Build history of the part. All positions in model axes, mm. Face numbers are marked on the shaded views. A direction names the side the tool comes from. Round coordinates to 2 decimals unless told otherwise and drop trailing zeros. Write each loop counter-clockwise with the first axis right and the second up, starting at its lowest first coordinate (ties: lowest second). Pieces come first, ordered by that corner, then holes. Notation, with made-up numbers: (-20.5, -14) - (0.5, -14) arc R30 ccw to (0.5, 9) - close; hole circle Ø11 at (46, 30.5). An arc over 180 degrees is marked (long way). One line per question, with ' | ' between items.
from build123d import *

# Parameters (mm, degrees)
F1_DEPTH = 76.2
F3_DEPTH = 25.4
F5_DEPTH = 49.022
F6_R     = 15.3034000689
F6_R_2   = 10.835787307
F6_R_3   = 5.9493654503
F7_DEPTH = 25.4
F8_DEPTH = 12.7
F9_DEPTH = 120.396


# Not quite as in the source:
# - a fillet or chamfer that OpenCascade refuses, or shapes differently, is made with other operations: its cross-section is extruded or revolved along the edge and cut away or added


with BuildPart() as f1:
    # F0 (on Front) → F1 (new body)
    with BuildSketch(Plane.XZ):
        Polygon((43.6695814133, 73.2915997505), (0, 0), (-37.7974100411, 0), (-75.9054422379, 48.224221915), (-75.9054422379, -55.3548447788), (43.6695814133, -55.3548447788), align=None)
    extrude(amount=F1_DEPTH)

    # F2 (on face) → F3 (join)
    with BuildSketch(Plane.XZ.offset(76.2)):
        Polygon((43.6695814133, 73.2915997505), (0, 0), (0, -55.3548447788), (43.6695814133, -55.3548447788), align=None)
    extrude(amount=F3_DEPTH)

    # F4 (on face) → F5 (cut)
    with BuildSketch(Plane.XZ.offset(76.2)):
        Polygon((-75.9054422379, 0), (-37.7974100411, 0), (-75.9054422379, 48.224221915), align=None)
    extrude(amount=-F5_DEPTH, mode=Mode.SUBTRACT)

    # F6 (on face) → F7 (join)
    with BuildSketch(Plane.XY):
        with Locations((-18.1702096015, -18.0441774428)):
            Circle(F6_R)
        with Locations((-44.1785492003, -40.8460125327)):
            Circle(F6_R_2)
        with Locations((-63.5862797499, -57.4966222048)):
            Circle(F6_R_3)
    extrude(amount=F7_DEPTH)

    # F8 (cut): a face of the model
    f8_faces = [f1.faces().sort_by_distance(p)[0] for p in [
        (-56.8514261395, -13.589, 24.1121109575),
    ]]
    extrude(f8_faces, amount=-F8_DEPTH, mode=Mode.SUBTRACT)

    # F9 (cut): a face of the model
    f9_faces = [f1.faces().sort_by_distance(p)[0] for p in [
        (-63.5862797499, -57.4966222048, 25.4),
    ]]
    extrude(f9_faces, amount=-F9_DEPTH, mode=Mode.SUBTRACT)

    # F10: fillet of radius 5.08 on 3 edges, made by hand

    # F10_s1 → F10_t2 (revolve, cut)
    with BuildSketch(Plane.XZ.offset(40.8460125327)):
        with BuildLine():
            ThreePointArc((-33.3427618933, 20.32), (-34.8306594448, 23.9121024484), (-38.4227618933, 25.4))
            Line((-38.4227618933, 25.4), (-33.3427618933, 25.4))
            Line((-33.3427618933, 25.4), (-33.3427618933, 20.32))
        make_face()
    revolve(axis=Axis((-44.1785492003, -40.8460125327, 25.4), (0, 0, 1)), mode=Mode.SUBTRACT)


with BuildPart() as f10_tool4:
    # F10_s5 → F10_t6 (revolve)
    with BuildSketch(Plane.XZ.offset(40.8460125327)):
        with BuildLine():
            ThreePointArc((-28.2627618933, 0), (-31.8548643417, 1.4878975516), (-33.3427618933, 5.08))
            Line((-33.3427618933, 5.08), (-33.3427618933, 0))
            Line((-33.3427618933, 0), (-28.2627618933, 0))
        make_face()
    revolve(axis=Axis((-44.1785492003, -40.8460125327, 0), (0, 0, 1)))

    split(bisect_by=Plane.XZ.offset(27.178), keep=Keep.TOP)


with BuildPart() as f1_1:
    add(f1.part)

    # F10_t3: union F10_tool4
    add(f10_tool4.part)


with BuildPart() as f10_tool9:
    # F10_s10 → F10_t11 (revolve)
    with BuildSketch(Plane.XZ.offset(40.8460125327)):
        with BuildLine():
            ThreePointArc((-28.2627618933, 0), (-31.8548643417, 1.4878975516), (-33.3427618933, 5.08))
            Line((-33.3427618933, 5.08), (-33.3427618933, 0))
            Line((-33.3427618933, 0), (-28.2627618933, 0))
        make_face()
    revolve(axis=Axis((-44.1785492003, -40.8460125327, 0), (0, 0, 1)))

    split(bisect_by=Plane(origin=(-14.5296914395, 0, 18.3867553359), x_dir=(0, 1, 0), z_dir=(0.6200078307, 0, -0.7845956218)), keep=Keep.TOP)


with BuildPart() as f1_2:
    add(f1_1.part)

    # F10_t8: union F10_tool9
    add(f10_tool9.part)

    # F11: chamfer of 5.08 on 3 edges, made by hand


with BuildPart() as f11_tool2:
    # F11_s3 → F11_t4 (revolve)
    with BuildSketch(Plane.XZ.offset(18.0441774428)):
        Polygon((2.2131904673, 0), (-2.8668095327, 5.08), (-2.8668095327, 0), align=None)
    revolve(axis=Axis((-18.1702096015, -18.0441774428, 0), (0, 0, 1)))

    split(bisect_by=Plane.XZ, keep=Keep.TOP)

    split(bisect_by=Plane(origin=(-14.5296914395, 0, 18.3867553359), x_dir=(0, 1, 0), z_dir=(0.6200078307, 0, -0.7845956218)), keep=Keep.TOP)


with BuildPart() as f1_3:
    add(f1_2.part)

    # F11_t1: union F11_tool2
    add(f11_tool2.part)

    # F11_s7 → F11_t8 (revolve, cut)
    with BuildSketch(Plane.XZ.offset(18.0441774428)):
        Polygon((-2.8668095327, 20.32), (-7.9468095327, 25.4), (-2.8668095327, 25.4), align=None)
    revolve(axis=Axis((-18.1702096015, -18.0441774428, 25.4), (0, 0, 1)), mode=Mode.SUBTRACT)


solid = f1_3.part
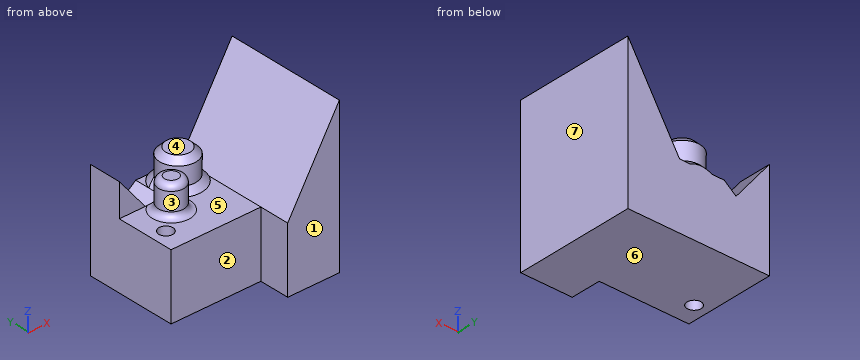
Q1. Drop flat-ended pins along their axis: pin 1 (1 mm diameter, centred on x = -37, y = -25, fed in from +Z); pin 2 (7 mm diameter, centred on x = -63.59, y = -57.5, fed in from -Z); pin 3 (6.5 mm diameter, centred on x = -67.5, z = 7.5, fed in from -Y); pin 4 (8 mm diameter, centred on x = -31, y = -7, fed in from +Z). Give the stop position or say it passes through.
Found:
pin 1: z = 0.81 | pin 2: through | pin 3: y = -27.18 | pin 4: z = 22.69
Q2. Drill centre lines: L1, parallel to X at y = -21, z = 2; L2, parallel to X at y = -84.5, z = -7.5; L3, parallel to X at y = -8.5, z = -4.5. Where is each one in solid material? Low to high. Write a range as from..to.
Found:
L1: -75.91..-55.56, -35.27..-0.03, 1.19..43.67 | L2: 0..43.67 | L3: -75.91..-50.43, -43.49..43.67
Q3. Saw through at B-B, the plane y = -78.5. List the corners of the cut face in (x, z), then the cut area to 3 significant figures.
Found:
outline: (0, -55.35) - (43.67, -55.35) - (43.67, 73.29) - (0, 0) - close | area: 4,020 mm^2
Q4. Pull direction X, two halves, no side cores. Call the marked faces 4, 5, 6 and 7: +X half, -X half, draft (parallel to the pull), parting line (faces both ways), or undercut.
Found:
face 4: undercut | face 5: undercut | face 6: draft | face 7: +X half
Q5. Saw through at C-C, the plane z = 57. List the corners of the cut face in (x, y), then the cut area to 3 significant figures.
Found:
outline: (33.96, -101.6) - (43.67, -101.6) - (43.67, 0) - (33.96, 0) - close | area: 986 mm^2
Q6. Saw through at A-A, the plane x = -63. List the corners of the cut face in (y, z).
Found:
outline: (-76.2, -55.35) - (-63.42, -55.35) - (-63.42, 0) - (-76.2, 0) - close; (-51.58, -55.35) - (0, -55.35) - (0, 11.41) - (-27.18, 11.41) - (-27.18, 0) - (-51.58, 0) - close
Q7. Which spindle directions (+Z, -Z, +X, -X, +Y, -Y) get a long thin tool onto all of the face, cutting with end or side? Do the marked faces 1, 2 and 3. Say none if no direction does.
Found:
face 1: +Z, -Z, +X, -X, -Y | face 2: +Z, -Z, -X, -Y | face 3: +Z
